Build history of the part. All positions in model axes, mm. Round coordinates to 2 decimals unless told otherwise and drop trailing zeros. Write each loop counter-clockwise with the first axis right and the second up, starting at its lowest first coordinate (ties: lowest second). Pieces come first, ordered by that corner, then holes. Notation, with made-up numbers: (-18, 65.5) - (1, 65.5) arc R11 cw to (1, 69.5) - close; hole circle Ø9 at (-31.5, 14.25). An arc over 180 degrees is marked (long way). One line per question, with ' | ' between items.
from build123d import *

# Parameters (mm, degrees)
EXTRUDE_1_DEPTH     = 5
SKETCH_3_W          = 1
SKETCH_3_H          = 224.141744844
CUT_EXTRUDE_2_DEPTH = 1
FILLET_1_R          = 10
SKETCH_7_R          = 1.5
CUT_EXTRUDE_3_DEPTH = 10


with BuildPart() as part:
    # 草图1 → 凸台-拉伸1 (new body)
    with BuildSketch(Plane.XY):
        Polygon((-172.5, 0), (172.5, 0), (76, -98.649632539), (-76, -98.649632539), align=None)
    extrude(amount=EXTRUDE_1_DEPTH)

    # 草图3 → 切除-拉伸2 (cut)
    with BuildSketch(Plane(origin=(0, 0, 0), x_dir=(-1, 0, 0), z_dir=(0, 0, -1))):
        with Locations((0, -49.835742657)):
            Rectangle(SKETCH_3_W, SKETCH_3_H)
    extrude(amount=-CUT_EXTRUDE_2_DEPTH, mode=Mode.SUBTRACT)

    # 圆角1
    # the kernel refuses this fillet: 10 mm, written as the material it takes off along each edge
    with BuildSketch(Plane(origin=(97.650635095, -98.649632539, 0), x_dir=(0, 1, 0), z_dir=(-1, 0, 0)), Plane(origin=(21.150635095, -98.649632539, 0), x_dir=(0, 1, 0), z_dir=(-1, 0, 0))) as fillet_1_piece_1:
        with BuildLine():
            CenterArc((8.660254038, -10), FILLET_1_R, 90, 60)
            Line((0, -5), (0, 0))
            Line((0, 0), (8.660254038, 0))
        make_face()
    extrude(amount=118.801270189, mode=Mode.SUBTRACT)

    # 草图7 → 切除-拉伸3 (cut)
    with BuildSketch(Plane(origin=(0, 0, 0), x_dir=(-1, 0, 0), z_dir=(0, 0, -1))):
        with Locations((55.2, -14.174704167)):
            Circle(SKETCH_7_R)
        with Locations((47.2, -14.174704167)):
            Circle(SKETCH_7_R)
        with Locations((47.2, -6.174704167)):
            Circle(SKETCH_7_R)
        with Locations((55.2, -6.174704167)):
            Circle(SKETCH_7_R)
        with Locations((-55.2, -6.174704167)):
            Circle(SKETCH_7_R)
        with Locations((-55.2, -14.174704167)):
            Circle(SKETCH_7_R)
        with Locations((-47.2, -14.174704167)):
            Circle(SKETCH_7_R)
        with Locations((-47.2, -6.174704167)):
            Circle(SKETCH_7_R)
    extrude(amount=-CUT_EXTRUDE_3_DEPTH, mode=Mode.SUBTRACT)


solid = part.part
Q1. Saw through at A-A, the plane z = 4.2. State how many separate pieces and enclosed holes the cut face has, then the cut area to 3 significant figures.
Found:
separate pieces: 1 | enclosed holes: 8 | area: 24,400 mm^2
Q2. Saw through at B-B, the plane y = -74. List the corners of the cut face in (x, z).
Found:
outline: (-100.11, 0) - (-0.5, 0) - (-0.5, 1) - (0.5, 1) - (0.5, 0) - (100.11, 0) - (100.11, 5) - (-100.11, 5) - close
Q3. Drill centre lines: L1, parallel to Y at x = 55.2, z = 1.35; L2, parallel to Y at x = -47.2, z = 1.75; L3, parallel to X at y = -44.5, z = 0.5. Where is each one in solid material? Low to high. Write a range as from..to.
Found:
L1: -95.01..-15.67, -12.67..-7.67, -4.67..0 | L2: -95.64..-15.67, -12.67..-7.67, -4.67..0 | L3: -128.97..-0.5, 0.5..128.97
Q4. Saw through at C-C, the plane x = 132. List the corners of the cut face in (y, z), then the cut area to 3 significant figures.
Found:
outline: (-41.4, 0) - (0, 0) - (0, 5) - (-41.4, 5) - close | area: 207 mm^2
Q5. Drop flat-ended pins along their axis: pin 1 (2.5 mm diameter, centred on x = 55.2, y = -6.17, fed in from -Z); pin 2 (1.1 mm diameter, centred on y = -24, z = 0.5, fed in from +X); pin 3 (0.5 mm diameter, centred on y = -51, z = 0.5, fed in from -X). Give the stop position or say it passes through.
Found:
pin 1: through | pin 2: x = 149.56 | pin 3: x = -122.86
Q6. Saw through at D-D, the plane y = -26.5. List the corners of the cut face in (x, z), then the cut area to 3 significant figures.
Found:
outline: (-146.58, 0) - (-0.5, 0) - (-0.5, 1) - (0.5, 1) - (0.5, 0) - (146.58, 0) - (146.58, 5) - (-146.58, 5) - close | area: 1,460 mm^2
